Could you check a few things on this model? Use its own coordinates, in mm. A direction names the side the tool comes from. Coordinates: 2 decimals unless noted, no trailing zeros. Order: outer loops, then holes, each group sorted by start corner. A loop starts at its lowest first (then second) coordinate and runs counter-clockwise, first axis right, second up. Notation, with made-up numbers: (29, 78.5) -> (48, 78.5) arc R22 ccw to (48, 115.5) -> close; hole circle Ø5 at (55.5, -29.5). An arc over 180 degrees is marked (long way). Use a Markdown table: item, result. Add a question column.
1) If I drill on L1, parallel to X at y = 2.75, z = -27; L2, parallel to X at y = 3.25, z = -85; L3, parallel to Z at x = -65, y = 2.7, over which ranges is the centre line in solid material (lowest first)? Write a range as [from, to].
2) Which directions (+Z, -Z, +X, -X, +Y, -Y) give clear straight access to the entire face, cutting with the end or side of a thin tool? Please do faces 1 (the flat face through (-12, 4, -91)), 2 (the flat face through (-24, 4, -92)), 3 (the cylindrical face through (-57.786, 4.578, -28.369)), 4 (the flat face through (-64, 4, -83.8)).
3) Thinking about a two-plate mould opening in Z: for faces 5 (the flat face through (-35, 4, -92)), 6 (the cylindrical face through (-6.488, 4.578, -87.196)), which applies, +Z half, -Z half, draft (parallel to the pull), parting line (faces both ways), or undercut?
4) If we section it at D-D (x = -65): Write out the boundary of the cut face in (y, z).
5) If we section it at C-C (z = -5): Write out the boundary of the cut face in (x, y).
6) Will these pins go through, and if not, where does the flat tip stop? pin 1 Ø5.5 at (x, z) = (-65, -5) entering from +Y; pin 2 Ø3 at (x, z) = (-32.5, -13.5) entering from +Y; pin 3 Ø0.6 at (x, y) = (-51, 3.5) entering from +Z; pin 4 Ø2 at (x, z) = (-6, -85) entering from +Y.
7) If we section it at A-A (z = -96): Write out the boundary of the cut face in (x, y), plus the area to 3 significant figures.
8) If we section it at B-B (x = -56): Write out the boundary of the cut face in (y, z), plus the area to 3 significant figures.
Autodesk Inventor part; units mm, degrees
ref_plane "YZ Plane" through (0, 0, 0) normal (1, 0, 0) x (0, 1, 0)
ref_plane "XZ Plane" through (0, 0, 0) normal (0, 1, 0) x (-1, 0, 0)
ref_plane "XY Plane" through (0, 0, 0) normal (0, 0, 1) x (1, 0, 0)
sketch "Sketch1" plane through (0, 0, 0) normal (0, 1, 0) x (-1, 0, 0)
  line L0 (0, 0) -> (59, 0)
  line L1 (59, 0) -> (59, -91)
  line L2 (59, -91) -> (0, -91)
  line L3 (0, -91) -> (0, 0)
  dimension "d0" = 59
  dimension "d1" = 91
extrude "Extrusion1" add sketch "Sketch1" along normal blind 3
sketch "Sketch2" plane through (0, 3, 0) normal (0, 1, 0) x (1, 0, 0)
  line L0 (0, 0) -> (-69, 0)
  line L1 (-69, 0) -> (-69, 101)
  line L2 (-69, 101) -> (0, 101)
  line L3 (0, 101) -> (0, 0)
  line L4 (-59, 91) -> (-59, 0)
  line L5 (0, 91) -> (-59, 91)
  dimension "d4" = 10
  dimension "d5" = 10
extrude "Extrusion2" add sketch "Sketch2" along normal blind 2 and the other way blind 3 contours L0 L1 L2 L3 L5 L4
sketch "Sketch3" plane through (0, 3, 0) normal (0, 1, 0) x (1, 0, 0)
  circle A0 centre (-56, 27) radius 1.35
  line L0 (-59, 0) -> (-59, 91)
  line L1 (-59, 0) -> (0, 0)
  circle A1 centre (-6, 27) radius 1.35
  line L2 (0, 0) -> (0, 91)
  circle A2 centre (-56, 85) radius 1.35
  line L3 (-59, 91) -> (0, 91)
  circle A3 centre (-6, 85) radius 1.35
  dimension "d10" = 2.7
  dimension "d11" = 3
  dimension "d12" = 27
  dimension "d13" = 2.7
  dimension "d14" = 6
  dimension "d15" = 27
  dimension "d16" = 2.7
  dimension "d17" = 3
  dimension "d18" = 6
  dimension "d19" = 2.7
  dimension "d20" = 6
  dimension "d21" = 6
extrude "Extrusion3" cut sketch "Sketch3" against normal blind 3 contours A0 | A1 | A2 | A3
sketch "Sketch4" plane through (0, 3, 0) normal (0, 1, 0) x (1, 0, 0)
  point P0 (0, 0)
sketch "Sketch5" plane through (0, 3, 0) normal (0, 1, 0) x (1, 0, 0)
  circle A0 centre (-56, 27) radius 2.25
  circle A1 centre (-56, 27) radius 1.35
  circle A2 centre (-56, 85) radius 2.25
  circle A3 centre (-6, 85) radius 2.25
  circle A4 centre (-6, 85) radius 1.35
  circle A5 centre (-56, 85) radius 1.35
  circle A6 centre (-6, 27) radius 2.25
  circle A7 centre (-6, 27) radius 1.35
  point P0 (0, 0)
  dimension "d24" = 0
  dimension "d25" = 0
  dimension "d26" = 4.5
  dimension "d27" = 4.5
  dimension "d28" = 4.5
  dimension "d29" = 0
  dimension "d30" = 0
  dimension "d31" = 0
  dimension "d32" = 4.5
  dimension "d33" = 0.9
  dimension "d34" = 0.9
  dimension "d35" = 0.9
  dimension "d36" = 0.9
extrude "Extrusion4" add sketch "Sketch5" along normal blind 3.2
sketch "Sketch6" plane through (-59, 3, -91) normal (0, 0, 1) x (1, 0, 0)
  line L0 (0, 2) -> (59, 2)
  line L1 (0, 0) -> (59, 0)
  line L2 (24, 2) -> (35, 2)
  line L3 (35, 2) -> (35, 0)
  line L4 (35, 0) -> (24, 0)
  line L5 (24, 0) -> (24, 2)
  line L6 (59, 0) -> (59, 2)
  line L7 (0, 0) -> (0, 2)
  point P0 (59, -3)
  point P1 (24, 0)
  dimension "d39" = 11
  dimension "d40" = 24
  dimension "d41" = 24
extrude "Extrusion5" cut sketch "Sketch6" against normal blind 3 contours L0 L3 L1 L5
sketch "Sketch7" plane through (0, 5, 0) normal (0, 1, 0) x (1, 0, 0)
  circle A0 centre (-65, 5) radius 1.75
  line L0 (-69, 101) -> (-69, 0)
  line L1 (-69, 0) -> (-59, 0)
  circle A1 centre (-65, 96) radius 1.75
  line L2 (0, 101) -> (-69, 101)
  circle A2 centre (-4, 96) radius 1.75
  line L3 (0, 91) -> (0, 101)
  point P0 (0, 0)
  dimension "d44" = 3.5
  dimension "d45" = 4
  dimension "d46" = 5
  dimension "d47" = 3.5
  dimension "d48" = 4
  dimension "d49" = 5
  dimension "d50" = 3.5
  dimension "d51" = 5
  dimension "d52" = 4
extrude "Extrusion6" cut sketch "Sketch7" against normal blind 19
sketch "Sketch8" plane through (0, 5, 0) normal (0, 1, 0) x (1, 0, 0)
  line L0 (-69, 101) -> (-69, 0)
  line L1 (-59, 83.8) -> (-69, 83.8)
  line L2 (-69, 83.8) -> (-69, 28.2)
  line L3 (-69, 28.2) -> (-59, 28.2)
  line L4 (-59, 28.2) -> (-59, 83.8)
  line L5 (-59, 0) -> (-59, 91)
  circle A0 centre (-56, 27) radius 2.25
  circle A1 centre (-56, 85) radius 1.35
  point P0 (0, 0)
  dimension "d55" = 0
  dimension "d56" = 1.2
  dimension "d57" = 1.2
extrude "Extrusion7" cut sketch "Sketch8" against normal blind 2 contours L1 L4 L3 L0
properties part number "ThridPrototypeRaspPiBed"
Answer sheet:
| question | item | result |
|---|---|---|
| 1 | L1 | [-69, -57.35], [-54.65, -7.35], [-4.65, 0] |
| 1 | L2 | [-69, -59], [-58.25, -57.35], [-54.65, -53.75], [-8.25, -7.35], [-4.65, -3.75] |
| 1 | L3 | [-101, -97.75], [-94.25, -6.75], [-3.25, 0] |
| 2 | face 1 | +X, +Y |
| 2 | face 2 | +Z, +Y |
| 2 | face 3 | +Y |
| 2 | face 4 | -X, +Y |
| 3 | face 5 | draft |
| 3 | face 6 | undercut |
| 4 | outline | (0, -101) -> (5, -101) -> (5, -97.75) -> (0, -97.75) -> close; (0, -94.25) -> (5, -94.25) -> (5, -83.8) -> (3, -83.8) -> (3, -28.2) -> (5, -28.2) -> (5, -6.75) -> (0, -6.75) -> close; (0, -3.25) -> (5, -3.25) -> (5, 0) -> (0, 0) -> close |
| 5 | outline | (-69, 0) -> (-66.75, 0) -> (-66.75, 5) -> (-69, 5) -> close; (-63.25, 0) -> (0, 0) -> (0, 3) -> (-59, 3) -> (-59, 5) -> (-63.25, 5) -> close |
| 6 | pin 1 | y = 5 |
| 6 | pin 2 | y = 3 |
| 6 | pin 3 | z = -91 |
| 6 | pin 4 | through |
| 7 | outline | (-69, 0) -> (-66.75, 0) -> (-66.75, 5) -> (-69, 5) -> close; (-63.25, 0) -> (-5.75, 0) -> (-5.75, 5) -> (-63.25, 5) -> close; (-2.25, 0) -> (0, 0) -> (0, 5) -> (-2.25, 5) -> close |
| 7 | area | 310 mm2 |
| 8 | outline | (0, -101) -> (5, -101) -> (5, -91) -> (3, -91) -> (3, -87.25) -> (6.2, -87.25) -> (6.2, -86.35) -> (0, -86.35) -> close; (0, -83.65) -> (6.2, -83.65) -> (6.2, -82.75) -> (3, -82.75) -> (3, -29.25) -> (6.2, -29.25) -> (6.2, -28.35) -> (0, -28.35) -> close; (0, -25.65) -> (6.2, -25.65) -> (6.2, -24.75) -> (3, -24.75) -> (3, 0) -> (0, 0) -> close |
| 8 | area | 318 mm2 |
